```python
from build123d import *

# Parameters (mm, degrees)
SKETCH_2_R          = 1.6
SKETCH_2_R_2        = 12.5
SKETCH_2_W          = 60
SKETCH_2_H          = 4
EXTRUDE_1_DEPTH     = 4
SKETCH_3_W          = 60
SKETCH_3_H          = 4
EXTRUDE_2_DEPTH     = 25
SKETCH_4_R          = 1.6
CUT_EXTRUDE_1_DEPTH = 25


with BuildPart() as part:
    # 草图2 → 凸台-拉伸1 (new body)
    # profile 1 of 2: a face of its own
    with BuildSketch(Plane.XY):
        Polygon((23.211946481, 19), (-16.788053519, 19), (-26.788053519, -21), (33.211946481, -21), align=None)
        with Locations((14.172101589, -10.960155108)):
            Circle(SKETCH_2_R, mode=Mode.SUBTRACT)
        with Locations((-7.748208627, -10.960155108)):
            Circle(SKETCH_2_R, mode=Mode.SUBTRACT)
        with Locations((-7.748208627, 10.960155108)):
            Circle(SKETCH_2_R, mode=Mode.SUBTRACT)
        with Locations((3.211946481, 0)):
            Circle(SKETCH_2_R_2, mode=Mode.SUBTRACT)
        with Locations((14.172101589, 10.960155108)):
            Circle(SKETCH_2_R, mode=Mode.SUBTRACT)
    # profile 2 of 2: a face of its own
    with BuildSketch(Plane.XY):
        with Locations((3.211946481, -23)):
            Rectangle(SKETCH_2_W, SKETCH_2_H)
    extrude(amount=EXTRUDE_1_DEPTH)

    # 草图3 → 凸台-拉伸2 (add)
    with BuildSketch(Plane(origin=(0, 0, 0), x_dir=(-1, 0, 0), z_dir=(0, 0, -1))):
        with Locations((-3.211946481, -23)):
            Rectangle(SKETCH_3_W, SKETCH_3_H)
    extrude(amount=EXTRUDE_2_DEPTH)

    # 草图4 → 切除-拉伸1 (cut)
    with BuildSketch(Plane.XZ.offset(25)):
        with Locations(Location((-21.788053519, -4.5, 0), (0, 0, 270))):
            Circle(SKETCH_4_R)
        with Locations(Location((28.211946481, -4.5, 0), (0, 0, 270))):
            Circle(SKETCH_4_R)
        with Locations(Location((28.211946481, -20.5, 0), (0, 0, 270))):
            Circle(SKETCH_4_R)
        with Locations(Location((-21.788053519, -20.5, 0), (0, 0, 270))):
            Circle(SKETCH_4_R)
    extrude(amount=-CUT_EXTRUDE_1_DEPTH, mode=Mode.SUBTRACT)


solid = part.part
```
Verification items for the finished model (mm, model axes). A direction names the side the tool comes from. Give positions to 0.01 mm unless a question says otherwise; leave off trailing zeros. Loops run counter-clockwise (first coordinate to the right, second up) from the corner with the lowest first, then second, coordinate; pieces in that order, holes last.
1. Section check B-B, the plane x = -22.5. Enter the section's corners in (y, z).
2. Section check D-D, the plane x = 1.5. Enter the section's corners in (y, z), then the cut area to 3 significant figures.
3. Go/stop test with flat-tipped pins: pin 1 Ø8 at (x, z) = (19, -21) entering from +Y; pin 2 Ø4 at (x, y) = (-8, 8) entering from -Z. Record where each tip stops, or that it passes through.
4. Set-up check for faces 4 (the flat face through (4, -21, -12)), 5 (the flat face through (28.28, -1.28, 1.97)): record each of +Z, -Z, +X, -X, +Y, -Y from which the full face is reachable in a straight line by a thin tool's end or side.
5. Section check A-A, the plane z = -20.5. Enter the section's corners in (x, y), then the cut area to 3 significant figures.
6. Section check C-C, the plane y = -2.5. Enter the section's corners in (x, z).
7. Thickness scan on line 1 (X direction, y = -23.3, z = -4.5); line 2 (Y direction, x = 3, z = 0.25); line 3 (Y direction, x = -21, z = -14.5). Record the ranges inside material, lowest first.
8. Mould release check, pull along Z, two halves, no side actions. Record for faces 1 (the cylindrical face through (27.6, -23.03, -5.98)), 2 (the flat face through (4, -23, -25)), 3 (the flat face through (33.212, -23, -10)): released by +Z, released by -Z, zero draft, split by the parting line, or undercut.
Geometry says:
1. outline: (-25, -25) - (-21, -25) - (-21, -21.93) - (-25, -21.93) - close; (-25, -19.07) - (-21, -19.07) - (-21, -5.93) - (-25, -5.93) - close; (-25, -3.07) - (-21, -3.07) - (-21, 0) - (-3.85, 0) - (-3.85, 4) - (-25, 4) - close
2. outline: (-25, -25) - (-21, -25) - (-21, 0) - (-12.38, 0) - (-12.38, 4) - (-25, 4) - close; (12.38, 0) - (19, 0) - (19, 4) - (12.38, 4) - close
2. area: 177 mm2
3. pin 1: stops at y = -21
3. pin 2: stops at z = 0
4. face 4: -Z, +X, -X, +Y
4. face 5: +Z, -Z, +X, +Y
5. outline: (-26.79, -25) - (-23.39, -25) - (-23.39, -21) - (-26.79, -21) - close; (-20.19, -25) - (26.61, -25) - (26.61, -21) - (-20.19, -21) - close; (29.81, -25) - (33.21, -25) - (33.21, -21) - (29.81, -21) - close
5. area: 214 mm2
6. outline: (-22.16, 0) - (-9.04, 0) - (-9.04, 4) - (-22.16, 4) - close; (15.46, 0) - (28.59, 0) - (28.59, 4) - (15.46, 4) - close
7. line 1: x = -26.79 to -23.39, -20.19 to 26.61, 29.81 to 33.21
7. line 2: y = -25 to -12.5, 12.5 to 19
7. line 3: y = -25 to -21
8. face 1: undercut
8. face 2: released by -Z
8. face 3: zero draft
